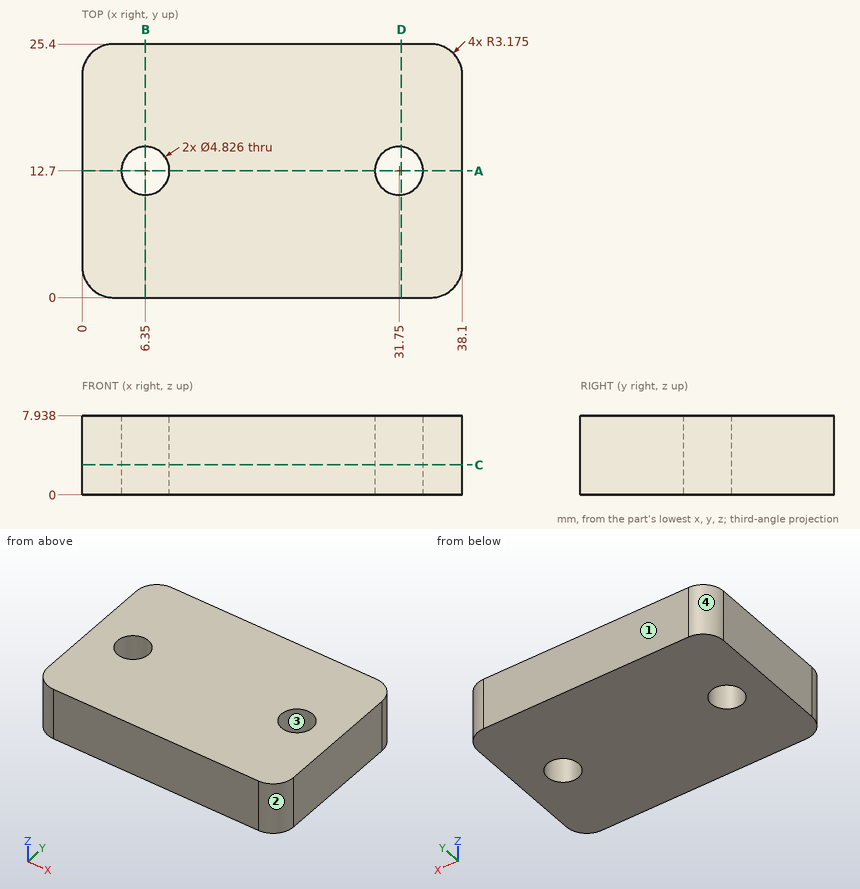
Design review of the part shown in the three views and the two pictorial views. Dimensions are in mm from the part's minimum x, y and z. Coordinates: 2 decimals unless noted, no trailing zeros. Order: outer loops, then holes, each group sorted by start corner. A loop starts at its lowest first (then second) coordinate and runs counter-clockwise, first axis right, second up.
Item 1: For line 1 (Y direction, x = 31.75, z = 3.25); line 2 (X direction, y = 12, z = 1.5); line 3 (X direction, y = 13.75, z = 2.25), list the stretches that pass through material, from the lowest coordinate up.
Item 2: Take a section at A-A, the plane y = 12.7. Write out the cut boundary in (x, z).
Item 3: Take a section at B-B, the plane x = 6.35. Write out the cut boundary in (y, z).
Item 4: Take a section at C-C, the plane z = 3. Count the separate pieces of the cut face and the enclosed holes in it.
Item 5: Take a section at D-D, the plane x = 32. Write out the cut boundary in (y, z).
Item 6: The part is to be moulded in two halves that separate along X. For the marked faces 1, 2, 3 and 4, say which applies: pulls with the +X half, pulls with the -X half, needs draft (parallel to the pull), parting line crosses it, or undercut.
The answers:
1. line 1: y = 0 to 10.29, 15.11 to 25.4
1. line 2: x = 0 to 4.04, 8.66 to 29.44, 34.06 to 38.1
1. line 3: x = 0 to 4.18, 8.52 to 29.58, 33.92 to 38.1
2. outline: (0, 0) - (3.94, 0) - (3.94, 7.94) - (0, 7.94) - close; (8.76, 0) - (29.34, 0) - (29.34, 7.94) - (8.76, 7.94) - close; (34.16, 0) - (38.1, 0) - (38.1, 7.94) - (34.16, 7.94) - close
3. outline: (0, 0) - (10.29, 0) - (10.29, 7.94) - (0, 7.94) - close; (15.11, 0) - (25.4, 0) - (25.4, 7.94) - (15.11, 7.94) - close
4. separate pieces: 1
4. enclosed holes: 2
5. outline: (0, 0) - (10.3, 0) - (10.3, 7.94) - (0, 7.94) - close; (15.1, 0) - (25.4, 0) - (25.4, 7.94) - (15.1, 7.94) - close
6. face 1: needs draft
6. face 2: pulls with the +X half
6. face 3: undercut
6. face 4: pulls with the -X half
